Geometry: final body of the model. Coordinates: model frame, mm. Face numbers are marked on the shaded views. A direction names the side the tool comes from. Give positions to 0.01 mm unless a question says otherwise; leave off trailing zeros. Write each loop counter-clockwise with the first axis right and the second up, starting at its lowest first coordinate (ties: lowest second). Pieces come first, ordered by that corner, then holes. Notation, with made-up numbers: M 44.25,73.5 L 67.25,73.5 A15 ccw 67.25,92.5 Z; hole C 83.5,65.5 d9. An arc over 180 degrees is marked long. Use one line per item in the form item = value. Start each with the question number.
Item 1: Contact query for flat-ended pins moving along their axis: P1, Ø1.8, axis at x = 6, z = 2, coming from the -Y side; P2, Ø2.5, axis at x = 9, y = 13.5, coming from the +Z side; P3, Ø12, axis at x = 17.5, z = 3.5, coming from the -Y side. Output: stop coordinate, or through.
Item 2: Section query B-B on z = 14. Return loops of the section in (x, y), then the cut area to 3 significant figures.
Item 3: Section query A-A on y = 14. Return loops of the section in (x, z).
Item 4: Access query for the marked faces 1, 2, 3 and 4. Directions: +Z, -Z, +X, -X, +Y, -Y. A direction counts if a zero-diameter tool reaches every point of the face in a straight line with its end or side. Return the directions, or none.
Item 5: Section query D-D on y = 5. Return loops of the section in (x, z), then the cut area to 3 significant figures.
Item 6: Section query C-C on x = 21. Return loops of the section in (y, z).
Item 7: Material intervals for line 1 along Y through (x, z) = (51.5, 3.1); line 2 along X through (y, z) = (11.75, 17.75); line 3 along Y through (x, z) = (50, 15), sorted ascending. Write a range as from..to.
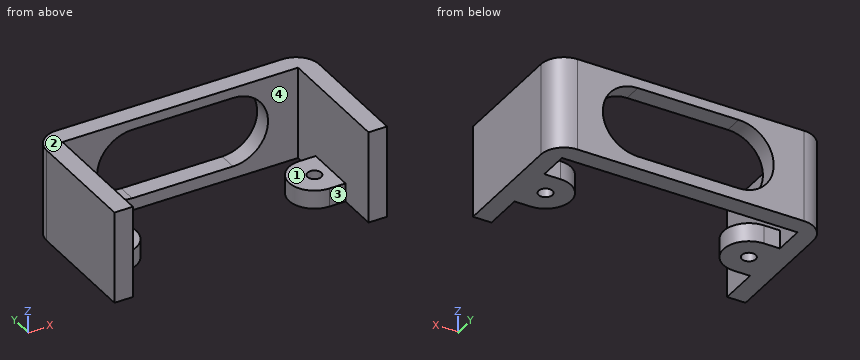
from build123d import *

# Parameters (mm, degrees)
SKETCH_1_R          = 1.5
EXTRUDE_1_DEPTH     = 4
EXTRUDE_1_2_DEPTH   = 4
EXTRUDE_2_DEPTH     = 20
FILLET_2_R          = 5
SKETCH_4_W          = 55
SKETCH_4_H          = 20
EXTRUDE_3_DEPTH     = 2
EXTRUDE_4_DEPTH     = 2
EXTRUDE_5_DEPTH     = 2
CUT_EXTRUDE_2_DEPTH = 7


with BuildPart() as part:
    # Sketch 1 → Extrude 1 (new body)
    with BuildSketch(Plane.XY):
        with BuildLine():
            Line((2, 19.5), (2, 8.5))
            Line((2, 8.5), (7.5, 8.5))
            ThreePointArc((7.5, 8.5), (13, 14), (7.5, 19.5))
            Line((7.5, 19.5), (2, 19.5))
        make_face()
        with Locations((7.5, 14)):
            Circle(SKETCH_1_R, mode=Mode.SUBTRACT)
    extrude(amount=EXTRUDE_1_DEPTH)



with BuildPart() as body_2:
    # Sketch 1 → Extrude 1 2 (new body)
    with BuildSketch(Plane.XY):
        with BuildLine():
            Line((51.5, 8.5), (57, 8.5))
            Line((57, 8.5), (57, 19.5))
            Line((57, 19.5), (51.5, 19.5))
            ThreePointArc((51.5, 19.5), (46, 14), (51.5, 8.5))
        make_face()
        with Locations((51.5, 14)):
            Circle(SKETCH_1_R, mode=Mode.SUBTRACT)
    extrude(amount=EXTRUDE_1_2_DEPTH)


with BuildPart() as part_1:
    add(part.part)

    add(body_2.part)  # Extrude 2 merges body 2
    # Sketch 1_3 → Extrude 2 (add)
    with BuildSketch(Plane.XY):
        Polygon((57, 28), (57, 0), (59, 0), (59, 30), (0, 30), (0, 0), (2, 0), (2, 28), align=None)
    extrude(amount=EXTRUDE_2_DEPTH)

    # Fillet 2
    fillet_2_edges = [part_1.edges().sort_by_distance(p)[0] for p in [
        (59, 30, 10),
        (0, 30, 10),
    ]]
    fillet(fillet_2_edges, radius=FILLET_2_R)

    # Sketch 4 → Extrude 3 (add)
    with BuildSketch(Plane.XZ.offset(-28)):
        with Locations((29.5, 10)):
            Rectangle(SKETCH_4_W, SKETCH_4_H)
    extrude(amount=EXTRUDE_3_DEPTH)

    # Sketch 5 → Extrude 4 (add)
    with BuildSketch(Plane(origin=(2, 0, 0), x_dir=(0, 0, -1), z_dir=(1, 0, 0))):
        Polygon((0, 8.5), (-4, 8.5), (-4, 19.5), (0, 19.5), (0, 26), (-20, 26), (-20, 0), (0, 0), align=None)
    extrude(amount=EXTRUDE_4_DEPTH)

    # Sketch 7 → Extrude 5 (add)
    with BuildSketch(Plane.ZY.offset(-57)):
        Polygon((0, 19.5), (4, 19.5), (4, 8.5), (0, 8.5), (0, 0), (20, 0), (20, 26), (0, 26), align=None)
    extrude(amount=EXTRUDE_5_DEPTH)

    # Sketch 8 → Cut-Extrude 2 (cut)
    with BuildSketch(Plane(origin=(0, 30, 0), x_dir=(1, 0, 0), z_dir=(0, 1, 0))):
        with BuildLine():
            Line((40.92, -17.832853898), (19.082552531, -17.832853898))
            ThreePointArc((19.082552531, -17.832853898), (11.500622297, -10.250923663), (19.082552531, -2.668993429))
            Line((19.082552531, -2.668993429), (40.92, -2.668993429))
            ThreePointArc((40.92, -2.668993429), (48.501930234, -10.250923663), (40.92, -17.832853898))
        make_face()
    extrude(amount=-CUT_EXTRUDE_2_DEPTH, mode=Mode.SUBTRACT)


solid = part_1.part
Answer sheet:
q1.P1 = 8.5
q1.P2 = 4
q1.P3 = 10.23
q2.outline = M 0,0 L 4,0 L 4,26 L 12.49,26 L 12.49,30 L 5,30 A5 ccw 0,25 Z; M 47.51,26 L 55,26 L 55,0 L 59,0 L 59,25 A5 ccw 54,30 L 47.51,30 Z
q2.area = 293 mm2
q3.outline = M 0,0 L 6,0 L 6,4 L 4,4 L 4,20 L 0,20 Z; M 9,0 L 13,0 L 13,4 L 9,4 Z; M 46,0 L 50,0 L 50,4 L 46,4 Z; M 53,0 L 59,0 L 59,20 L 55,20 L 55,4 L 53,4 Z
q4.face_1 = +Z, -Y
q4.face_2 = +Z, +X, -X, +Y, -Y
q4.face_3 = +Z, -Z, -Y
q4.face_4 = +Z, -Z
q5.outline = M 0,0 L 4,0 L 4,20 L 0,20 Z; M 55,0 L 59,0 L 59,20 L 55,20 Z
q5.area = 160 mm2
q6.outline = M 26,0 L 30,0 L 30,2.67 L 26,2.67 Z; M 26,17.83 L 30,17.83 L 30,20 L 26,20 Z
q7.line_1 = 8.5..12.5, 15.5..19.5, 26..30
q7.line_2 = 0..4, 55..59
q7.line_3 = 26..30
